Geometry: final body of the model. Coordinates: model frame, mm. A direction names the side the tool comes from. Coordinates: 2 decimals unless noted, no trailing zeros. Order: outer loops, then holes, each group sorted by start corner. A loop starts at its lowest first (then second) coordinate and runs counter-clockwise, first axis right, second up. Notation, with made-up numbers: M 73,30.5 L 88,30.5 A18 ccw 88,37.5 Z; hole C -5.5,89 d1. An arc over 180 degrees is marked long. Write item = value, one per line.
from build123d import *

# Parameters (mm, degrees)
SKETCH_1_W          = 60
SKETCH_1_H          = 24.832992812
SKETCH_1_R          = 2.2
EXTRUDE_2_DEPTH     = 2
SKETCH_6_W          = 2
SKETCH_6_H          = 22.832992812
SKETCH_6_W_2        = 60
SKETCH_6_H_2        = 2
EXTRUDE_3_DEPTH     = 30
CUT_EXTRUDE_1_DEPTH = 55.241767882
SKETCH_9_R          = 2.5
CUT_EXTRUDE_2_DEPTH = 51.405133984


with BuildPart() as part:
    # 草圖1 → 填料-伸長2 (new body)
    with BuildSketch(Plane(origin=(0, 0, 0), x_dir=(1, 0, 0), z_dir=(0, 1, 0))):
        Rectangle(SKETCH_1_W, SKETCH_1_H)
        with Locations(Location((-24.25, 0, 0), (0, 0, 270))):
            Circle(SKETCH_1_R, mode=Mode.SUBTRACT)
        with Locations(Location((0, 0, 0), (0, 0, 270))):
            Circle(SKETCH_1_R, mode=Mode.SUBTRACT)
        with Locations(Location((24.25, 0, 0), (0, 0, 270))):
            Circle(SKETCH_1_R, mode=Mode.SUBTRACT)
    extrude(amount=EXTRUDE_2_DEPTH)

    # 草圖6 → 填料-伸長3 (add)
    with BuildSketch(Plane(origin=(0, 2, 0), x_dir=(1, 0, 0), z_dir=(0, 1, 0))):
        with Locations((-11, 1)):
            Rectangle(SKETCH_6_W, SKETCH_6_H)
        with Locations((0, -11.416496406)):
            Rectangle(SKETCH_6_W_2, SKETCH_6_H_2)
        with Locations((11, 1)):
            Rectangle(SKETCH_6_W, SKETCH_6_H)
    extrude(amount=EXTRUDE_3_DEPTH)

    # 草圖8 → 除料-伸長1 (cut, through all)
    with BuildSketch(Plane.ZY.offset(12)):
        Polygon((10.416496406, 32), (-12.416496406, 2), (-12.416496406, 32), align=None)
    extrude(amount=-CUT_EXTRUDE_1_DEPTH, mode=Mode.SUBTRACT)

    # 草圖9 → 除料-伸長2 (cut, through all)
    with BuildSketch(Plane.XY.offset(12.416496406)):
        with Locations((-24.25, 13)):
            Circle(SKETCH_9_R)
        with Locations((24.25, 13)):
            Circle(SKETCH_9_R)
        with Locations((24.25, 23)):
            Circle(SKETCH_9_R)
        with Locations((-24.25, 23)):
            Circle(SKETCH_9_R)
    extrude(amount=-CUT_EXTRUDE_2_DEPTH, mode=Mode.SUBTRACT)


solid = part.part
1) Set-up query: faces 5 (the face through (21, 17, 10.416)), 6 (the face through (-30, 9, 11)), 7 (the face through (-10, 13, 2)), 8 (the face through (-21, 17, 10.416)). Return all of +Z, -Z, +X, -X, +Y, -Y with unobstructed straight access to the full face (end or side cutting, diameter ignored); none if empty.
Numbers:
face_5 = -Z, +X, +Y
face_6 = +Z, -Z, -X, +Y, -Y
face_7 = -Z, +Y
face_8 = -Z, -X, +Y
2) Section A-A, the plane x = 0. Return loops of the section in (y, z), and give its area (3 significant figures).
Numbers:
outline = M 0,-12.42 L 2,-12.42 L 2,-2.2 L 0,-2.2 Z; M 0,2.2 L 2,2.2 L 2,10.42 L 32,10.42 L 32,12.42 L 0,12.42 Z
area = 101 mm²
3) Section C-C, the plane y = 23. Return loops of the section in (x, z), and give its area (3 significant figures).
Numbers:
outline = M -30,10.42 L -26.75,10.42 L -26.75,12.42 L -30,12.42 Z; M -21.75,10.42 L -12,10.42 L -12,3.57 L -10,3.57 L -10,10.42 L 10,10.42 L 10,3.57 L 12,3.57 L 12,10.42 L 21.75,10.42 L 21.75,12.42 L -21.75,12.42 Z; M 26.75,10.42 L 30,10.42 L 30,12.42 L 26.75,12.42 Z
area = 127 mm²
4) Section D-D, the plane z = 0. Return loops of the section in (x, y), and give its area (3 significant figures).
Numbers:
outline = M -30,0 L -26.45,0 L -26.45,2 L -30,2 Z; M -22.05,0 L -2.2,0 L -2.2,2 L -10,2 L -10,18.31 L -12,18.31 L -12,2 L -22.05,2 Z; M 2.2,0 L 22.05,0 L 22.05,2 L 12,2 L 12,18.31 L 10,18.31 L 10,2 L 2.2,2 Z; M 26.45,0 L 30,0 L 30,2 L 26.45,2 Z
area = 159 mm²
5) Line query: L1, parallel to X at y = 0.55, z = 0; L2, parallel to X at y = 4.5, z = 9.25; L3, parallel to Z at x = 4, y = 19. Output: solid intervals per line, ascending.
Numbers:
L1 = -30 to -26.45, -22.05 to -2.2, 2.2 to 22.05, 26.45 to 30
L2 = -12 to -10, 10 to 12
L3 = 10.42 to 12.42
6) Mould query, pull axis X, two halves, no side actions, for faces 1 (the face through (22.102, 0.986, -0.477)), 2 (the face through (-26.09, 24.69, 11.43)), 3 (the face through (-11, 17, -1)), 4 (the face through (-12, 13, 2)). Classes: pulls with the +X half, pulls with the -X half, needs draft (parallel to the pull), parting line crosses it, or undercut.
Numbers:
face_1 = undercut
face_2 = undercut
face_3 = needs draft
face_4 = pulls with the -X half
7) Pin query (flat end, axial travel): pin 1 (6 mm diameter, centred on x = 3, y = 22.5, fed in from -Z); pin 2 (1.5 mm diameter, centred on x = -20.5, z = 1, fed in from +Y); pin 3 (4 mm diameter, centred on y = 4.5, z = -8, fed in from -X). Return the tip coordinate at first contact, or that it passes through.
Numbers:
pin_1 = 10.42
pin_2 = 2
pin_3 = -12
8) Section B-B, the plane x = -24.25. Return loops of the section in (y, z), and give its area (3 significant figures).
Numbers:
outline = M 0,-12.42 L 2,-12.42 L 2,-2.2 L 0,-2.2 Z; M 0,2.2 L 2,2.2 L 2,10.42 L 10.5,10.42 L 10.5,12.42 L 0,12.42 Z; M 15.5,10.42 L 20.5,10.42 L 20.5,12.42 L 15.5,12.42 Z; M 25.5,10.42 L 32,10.42 L 32,12.42 L 25.5,12.42 Z
area = 80.9 mm²
